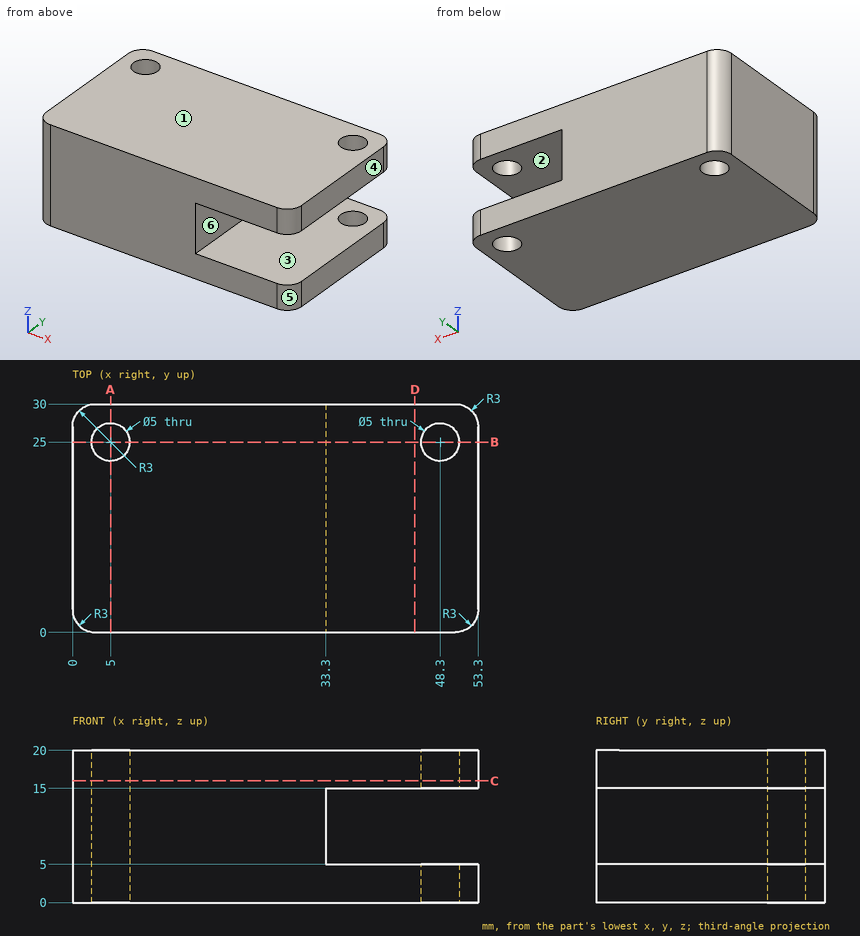
Print and shaded views of the part. All mm, measured from the part's lowest x, y and z. A direction names the side the tool comes from. Give positions to 0.01 mm unless a question says otherwise; leave off trailing zeros. Order: outer loops, then holes, each group sorted by start corner. A loop starts at its lowest first (then second) coordinate and runs counter-clockwise, first axis right, second up. Notation, with made-up numbers: (29.25, -23.75) -> (66.25, -23.75) arc R8 ccw to (66.25, -15.75) -> close; hole circle Ø4 at (0.25, 10). An arc over 180 degrees is marked (long way). Use CSV: the item, a comma, the result in double quotes.
1. 3-axis set-ups, long thin cutter, end or side, ignore diameter. For the marked faces 5 and 6: which of +Z, -Z, +X, -X, +Y, -Y reach the whole face in a straight line?
Outcome:
face 5,"+Z, -Z, +X, -Y"
face 6,"+X, +Y, -Y"
2. Mould opens along Z. For the marked faces 1, 2, 3 and 4 say: +Z half, -Z half, draft (parallel to the pull), parting line (faces both ways), or undercut.
Outcome:
face 1,"+Z half"
face 2,"undercut"
face 3,"undercut"
face 4,"draft"
3. Band-saw the part on A-A, the plane x = 5. Give the cut face in (y, z).
Outcome:
outline,"(0, 0) -> (22.5, 0) -> (22.5, 20) -> (0, 20) -> close; (27.5, 0) -> (30, 0) -> (30, 20) -> (27.5, 20) -> close"
4. Band-saw the part on C-C, the plane z = 16. Give the cut face in (x, y), then the cut area to 3 significant figures.
Outcome:
outline,"(0, 3) arc R3 ccw to (3, 0) -> (50.3, 0) arc R3 ccw to (53.3, 3) -> (53.3, 27) arc R3 ccw to (50.3, 30) -> (3, 30) arc R3 ccw to (0, 27) -> close; hole circle Ø5 at (5, 25); hole circle Ø5 at (48.3, 25)"
area,"1,550 mm²"
5. Drill centre lines: line 1 along Z through (x, y) = (49, 17.25); line 2 along X through (y, z) = (24.75, 7.75); line 3 along Y through (x, z) = (48.3, 2.1). Where is each one in solid material? Low to high. Write a range as from..to.
Outcome:
line 1,"0..5, 15..20"
line 2,"0..2.51, 7.49..33.3"
line 3,"0..22.5, 27.5..30"
6. Band-saw the part on D-D, the plane x = 45. Give the cut face in (y, z), then the cut area to 3 significant figures.
Outcome:
outline,"(0, 0) -> (30, 0) -> (30, 5) -> (0, 5) -> close; (0, 15) -> (30, 15) -> (30, 20) -> (0, 20) -> close"
area,"300 mm²"
7. Drop flat-ended pins along their axis: pin 1 (4.5 mm diameter, centred on x = 5, y = 25, fed in from +Z); pin 2 (12 mm diameter, centred on x = 43.5, y = 22.5, fed in from -Z). Give the stop position or say it passes through.
Outcome:
pin 1,"through"
pin 2,"z = 0"
8. Band-saw the part on B-B, the plane y = 25. Give the cut face in (x, z), then the cut area to 3 significant figures.
Outcome:
outline,"(0, 0) -> (2.5, 0) -> (2.5, 20) -> (0, 20) -> close; (7.5, 0) -> (45.8, 0) -> (45.8, 5) -> (33.3, 5) -> (33.3, 15) -> (45.8, 15) -> (45.8, 20) -> (7.5, 20) -> close; (50.8, 0) -> (53.3, 0) -> (53.3, 5) -> (50.8, 5) -> close; (50.8, 15) -> (53.3, 15) -> (53.3, 20) -> (50.8, 20) -> close"
area,"716 mm²"
